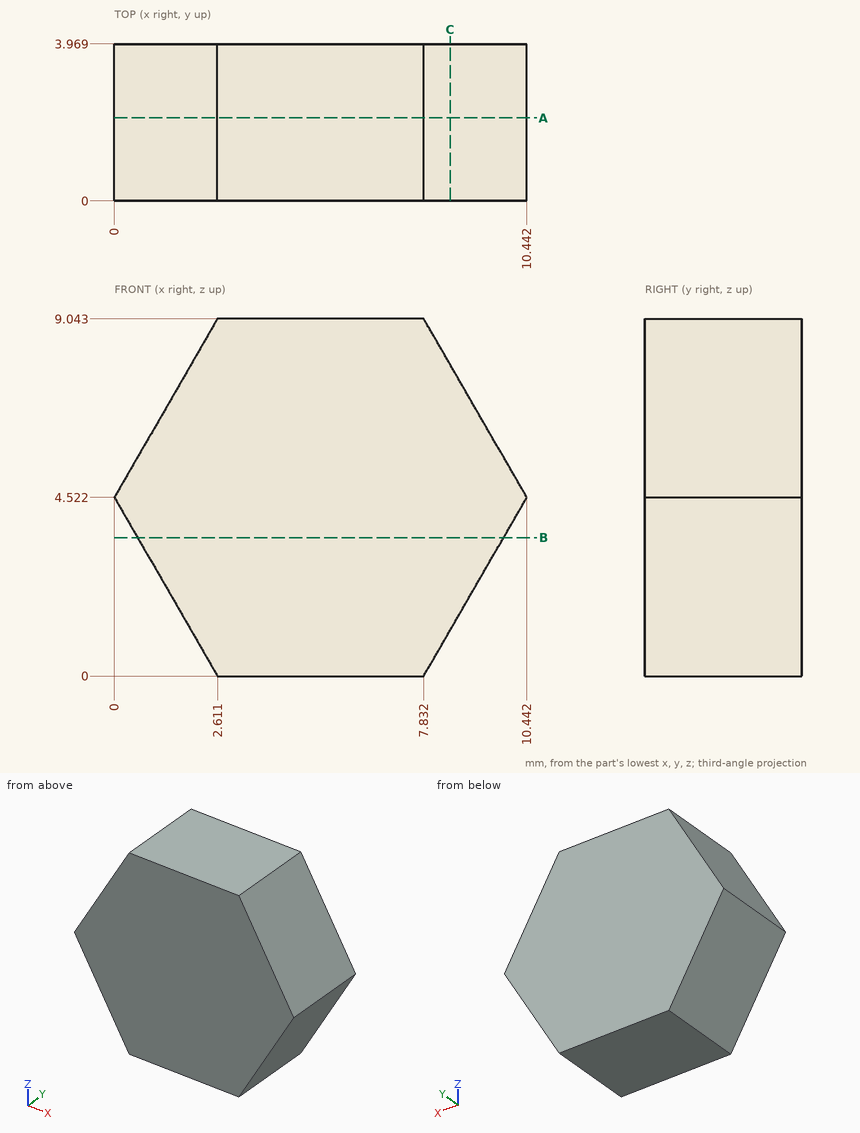
Check sheet for the drawn part. Datum: minimum x, y, z corner. Units: mm. Round coordinates to 2 decimals unless told otherwise and drop trailing zeros. Order: outer loops, then holes, each group sorted by start corner. A loop starts at its lowest first (then second) coordinate and runs counter-clockwise, first axis right, second up.
(1) Cross-section at A-A, the plane y = 2.1. Enter the section's corners in (x, z).
(2) Cross-section at B-B, the plane z = 3.5. Enter the section's corners in (x, y).
(3) Cross-section at C-C, the plane x = 8.5. Enter the section's corners in (y, z) (1 decimal), and give its area (3 significant figures).
(4) Go/stop test with flat-tipped pins: P1, Ø1.5, axis at y = 2, z = 3.5, coming from the +X side (1 decimal); P2, Ø1, axis at y = 2.5, z = 4, coming from the +X side. Record where each tip stops, or that it passes through.
(5) Scan lines: probe 1 along X at (y, z) = (2.6, 7.75) (1 decimal); probe 2 along Z at (x, y) = (1.5, 3) (1 decimal); probe 3 along X at (y, z) = (0.9, 7.5). Record each from-to range of solid material in increasing order.
Check sheet entries:
1. outline: (0, 4.52) - (2.61, 0) - (7.83, 0) - (10.44, 4.52) - (7.83, 9.04) - (2.61, 9.04) - close
2. outline: (0.59, 0) - (9.85, 0) - (9.85, 3.97) - (0.59, 3.97) - close
3. outline: (0, 1.2) - (4, 1.2) - (4, 7.9) - (0, 7.9) - close
3. area: 26.7 mm2
4. P1: stops at x = 10.3
4. P2: stops at x = 10.43
5. probe 1: x = 1.9 to 8.6
5. probe 2: z = 1.9 to 7.1
5. probe 3: x = 1.72 to 8.72
